Input: part model. Units: mm. Frame: model coordinates. A direction names the side the tool comes from. Round coordinates to 2 decimals unless told otherwise and drop trailing zeros. Order: outer loops, then holes, each group sorted by start corner. A loop starts at its lowest first (then second) coordinate and runs counter-clockwise, first axis right, second up. Notation, with made-up numbers: M 65,46 L 72,46 A20 cw 72,82 Z; hole C -8.5,76.25 d8. An arc over 180 degrees is marked long. One line per question, with ' | ' between items.
Autodesk Fusion 360 part; units mm, degrees
sketch "Sketch1" plane through (0, 0, 0) normal (0, 0, 1) x (1, 0, 0)
  line L0 (0, 0) -> (95.25, 0)
  line L1 (95.25, 0) -> (95.25, 95.25)
  line L2 (95.25, 95.25) -> (0, 95.25)
  line L3 (0, 95.25) -> (0, 0)
  dimension "d1" = 95.25
  dimension "d2" = 95.25
extrude "Extrude1" add sketch "Sketch1" along normal blind 3.2
sketch "Sketch2" plane through (0, 0, 3.2) normal (0, 0, 1) x (-1, 0, 0)
  line L0 (0, -95.25) -> (0, 0)
  line L1 (0, 0) -> (-95.25, 0)
  line L2 (-95.25, 0) -> (-95.25, -95.25)
  line L3 (-95.25, -95.25) -> (0, -95.25)
  circle A0 centre (-47.625, -47.625) radius 33
  circle A1 centre (-47.625, -47.625) radius 37
  line L4 (-23.4439, -57.8934) -> (-23.4439, -65.8934)
  line L5 (-23.4439, -65.8934) -> (-71.4439, -65.8934)
  line L6 (-71.4439, -65.8934) -> (-71.4439, -57.8934)
  line L7 (-42.3445, -22.9899) -> (-52.3445, -22.9899)
  line L8 (-52.3445, -22.9899) -> (-52.3445, -57.8934)
  line L9 (-42.3445, -57.8934) -> (-42.3445, -22.9899)
  line L10 (-71.4439, -57.8934) -> (-52.3445, -57.8934)
  line L11 (-42.3445, -57.8934) -> (-23.4439, -57.8934)
  point P0 (-47.625, -68.4053)
  point P1 (-47.625, -47.625)
  dimension "d5" = 66
  dimension "d6" = 4
  dimension "d9" = 48
  dimension "d10" = 8
fillet "Fillet1" radius 4 1 edges at (0, 0, 1.6)
fillet "Fillet2" radius 4 1 edges at (95.25, 0, 1.6)
fillet "Fillet3" radius 4 1 edges at (95.25, 95.25, 1.6)
fillet "Fillet4" radius 4 1 edges at (0, 95.25, 1.6)
extrude "Extrude2" add sketch "Sketch2" along normal blind 0.1 contours A1 | L4 L5 L6 L7 L8 L9 L10 L11
extrude "Extrude3" cut 1 faces at (59.86, 36.6396, 3.2) along direction (0, 0, -1) blind 0.01
extrude "Extrude4" cut 1 faces at (59.86, 36.6396, 3.19) along direction (0, 0, -1) blind 0.01
Item 1: Mould query, pull axis Y, two halves, no side actions, for faces 3 (the flat face through (54, 48, 3.18)), 4 (the flat face through (48, 54, 3.3)), 5 (the cylindrical face through (94.109, 94.047, 1.622)). Classes: +Y half, -Y half, draft (parallel to the pull), parting line (faces both ways), or undercut.
Report:
face 3: undercut | face 4: draft | face 5: +Y half
Item 2: Section query C-C, the plane x = 75.5. Return loops of the section in (y, z), plus the area to 3 significant figures.
Report:
outline: M 0,0 L 95.25,0 L 95.25,3.2 L 71.96,3.2 L 71.96,3.3 L 65.29,3.3 L 65.29,3.18 L 29.96,3.18 L 29.96,3.3 L 23.29,3.3 L 23.29,3.2 L 0,3.2 Z | area: 305 mm²
Item 3: Access query for faces 1 (the flat face through (81, 47, 3.3)), 2 (the flat face through (68, 80, 3.2)). Directions: +Z, -Z, +X, -X, +Y, -Y. A direction counts if a zero-diameter tool reaches every point of the face in a straight line with its end or side. Return the directions, or none.
Report:
face 1: +Z, +X, -X, +Y, -Y | face 2: +Z
Item 4: Section query B-B, the plane x = 31.5. Return loops of the section in (y, z), plus the area to 3 significant figures.
Report:
outline: M 0,0 L 95.25,0 L 95.25,3.2 L 80.93,3.2 L 80.93,3.3 L 76.42,3.3 L 76.42,3.18 L 65.89,3.18 L 65.89,3.3 L 57.89,3.3 L 57.89,3.18 L 18.83,3.18 L 18.83,3.3 L 14.32,3.3 L 14.32,3.2 L 0,3.2 Z | area: 306 mm²
Item 5: Line query: line 1 along Z through (x, y) = (36, 38.5). Output: solid intervals per line, ascending. Write a range as from..to.
Report:
line 1: 0..3.18
Item 6: Section query A-A, the plane y = 21.5. Return loops of the section in (x, z), plus the area to 3 significant figures.
Report:
outline: M 0,0 L 95.25,0 L 95.25,3.2 L 73.83,3.2 L 73.83,3.3 L 67.79,3.3 L 67.79,3.18 L 27.46,3.18 L 27.46,3.3 L 21.42,3.3 L 21.42,3.2 L 0,3.2 Z | area: 305 mm²
Item 7: Section query D-D, the plane y = 83.5. Return loops of the section in (x, z), plus the area to 3 significant figures.
Report:
outline: M 0,0 L 95.25,0 L 95.25,3.2 L 56.68,3.2 L 56.68,3.3 L 38.57,3.3 L 38.57,3.2 L 0,3.2 Z | area: 307 mm²
